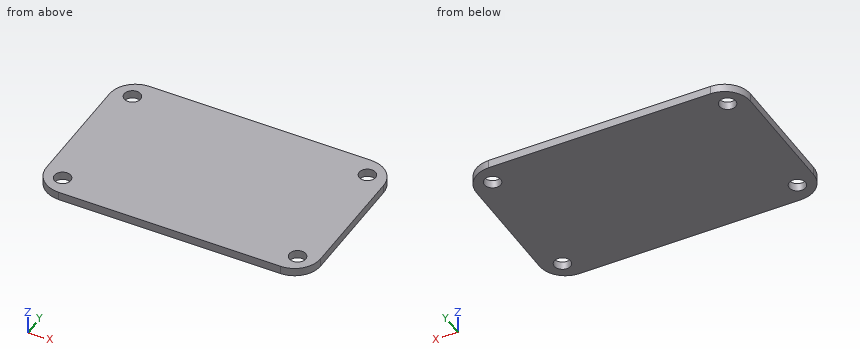
from build123d import *

# Parameters (mm, degrees)
BOSS_EXTRUDE1_DEPTH = 1.6002
SKETCH2_R           = 1.5875
CUT_EXTRUDE1_DEPTH  = 11.7602


with BuildPart() as part:
    # Sketch1 → Boss-Extrude1 (new body)
    with BuildSketch(Plane.XY):
        with BuildLine():
            Line((-21.59, 16.51), (21.59, 16.51))
            ThreePointArc((21.59, 16.51), (25.182102448, 15.022102448), (26.67, 11.43))
            Line((26.67, 11.43), (26.67, -11.43))
            ThreePointArc((26.67, -11.43), (25.182102448, -15.022102448), (21.59, -16.51))
            Line((21.59, -16.51), (-21.59, -16.51))
            ThreePointArc((-21.59, -16.51), (-25.182102448, -15.022102448), (-26.67, -11.43))
            Line((-26.67, -11.43), (-26.67, 11.43))
            ThreePointArc((-26.67, 11.43), (-25.182102448, 15.022102448), (-21.59, 16.51))
        make_face()
    extrude(amount=-BOSS_EXTRUDE1_DEPTH)

    # Sketch2 → Cut-Extrude1 (cut)
    with BuildSketch(Plane.XY):
        with Locations((-22.86, 12.7)):
            Circle(SKETCH2_R)
        with Locations((-22.86, -12.7)):
            Circle(SKETCH2_R)
        with Locations((22.86, 12.7)):
            Circle(SKETCH2_R)
        with Locations((22.86, -12.7)):
            Circle(SKETCH2_R)
    extrude(amount=-CUT_EXTRUDE1_DEPTH, mode=Mode.SUBTRACT)


solid = part.part
Part model, mm, in its own coordinate system. Coordinates: 2 decimals unless noted, no trailing zeros. Loops run counter-clockwise (first coordinate to the right, second up) from the corner with the lowest first, then second, coordinate; pieces in that order, holes last. Notation, with made-up numbers: (77.25, 41.5) -> (88.25, 41.5) arc R25 ccw to (88.25, 75.5) -> close; hole circle Ø7 at (-16.75, 12). An arc over 180 degrees is marked (long way). Use a Markdown table: item, result. Add a question column.
Item 1: Band-saw the part on C-C on y = 12.7. Write the cut outline in (x, z).
Item 2: Flat gauge pin, fed straight in: P1, Ø3, axis at x = -0.5, y = 6, coming from the +Z side. Where does the tip first touch, or does it go through?
Item 3: Band-saw the part on B-B on x = 22.86. Write the cut outline in (y, z), plus the area to 3 significant figures.
Item 4: Probe probe 1 along Y at (x, z) = (22.86, -1); probe 2 along X at (y, z) = (11.5, -0.7); probe 3 along X at (y, z) = (13, -1.5). List the from-to ranges inside material, lowest first.
Item 5: Band-saw the part on A-A on z = -0.6. Write the cut outline in (x, y) (1 decimal).
Geometry says:
| question | item | result |
|---|---|---|
| 1 | outline | (-26.51, -1.6) -> (-24.45, -1.6) -> (-24.45, 0) -> (-26.51, 0) -> close; (-21.27, -1.6) -> (21.27, -1.6) -> (21.27, 0) -> (-21.27, 0) -> close; (24.45, -1.6) -> (26.51, -1.6) -> (26.51, 0) -> (24.45, 0) -> close |
| 2 | P1 | z = 0 |
| 3 | outline | (-16.35, -1.6) -> (-14.29, -1.6) -> (-14.29, 0) -> (-16.35, 0) -> close; (-11.11, -1.6) -> (11.11, -1.6) -> (11.11, 0) -> (-11.11, 0) -> close; (14.29, -1.6) -> (16.35, -1.6) -> (16.35, 0) -> (14.29, 0) -> close |
| 3 | area | 42.2 mm² |
| 4 | probe 1 | -16.35 to -14.29, -11.11 to 11.11, 14.29 to 16.35 |
| 4 | probe 2 | -26.67 to -23.9, -21.82 to 21.82, 23.9 to 26.67 |
| 4 | probe 3 | -26.42 to -24.42, -21.3 to 21.3, 24.42 to 26.42 |
| 5 | outline | (-26.7, -11.4) arc R5.1 ccw to (-21.6, -16.5) -> (21.6, -16.5) arc R5.1 ccw to (26.7, -11.4) -> (26.7, 11.4) arc R5.1 ccw to (21.6, 16.5) -> (-21.6, 16.5) arc R5.1 ccw to (-26.7, 11.4) -> close; hole circle Ø3.2 at (-22.9, -12.7); hole circle Ø3.2 at (-22.9, 12.7); hole circle Ø3.2 at (22.9, -12.7); hole circle Ø3.2 at (22.9, 12.7) |
